The model under review builds one solid part; all positions refer to its coordinate system, in mm. A direction names the side the tool comes from. Round coordinates to 2 decimals unless told otherwise and drop trailing zeros. Loops run counter-clockwise (first coordinate to the right, second up) from the corner with the lowest first, then second, coordinate; pieces in that order, holes last. Notation, with made-up numbers: (77.25, -6.75) - (125.25, -6.75) arc R20 cw to (125.25, 22.25) - close; hole circle Ø7 at (-18, 13.5). An arc over 180 degrees is marked (long way). Answer as CSV lines item,"result".
from build123d import *

# Parameters (mm, degrees)
SKETCH1_W           = 177.8
SKETCH1_H           = 25.4
SKETCH1_W_2         = 167.64
SKETCH1_H_2         = 15.24
BOSS_EXTRUDE2_DEPTH = 25.4
SKETCH3_W           = 193.04
SKETCH3_H           = 39.37
SKETCH3_W_2         = 177.8
SKETCH3_H_2         = 25.4
BOSS_EXTRUDE3_DEPTH = 12.7


with BuildPart() as part:
    # Sketch1 → Boss-Extrude2 (new body)
    with BuildSketch(Plane.XY):
        with Locations((88.9, 12.7)):
            Rectangle(SKETCH1_W, SKETCH1_H)
        with Locations((88.9, 12.7)):
            Rectangle(SKETCH1_W_2, SKETCH1_H_2, mode=Mode.SUBTRACT)
    extrude(amount=BOSS_EXTRUDE2_DEPTH)

    # Sketch3 → Boss-Extrude3 (add)
    with BuildSketch(Plane.XY.offset(25.4)):
        with Locations((88.9, 14.605)):
            Rectangle(SKETCH3_W, SKETCH3_H)
        with Locations((88.9, 12.7)):
            Rectangle(SKETCH3_W_2, SKETCH3_H_2, mode=Mode.SUBTRACT)
    extrude(amount=-BOSS_EXTRUDE3_DEPTH)


solid = part.part
1. Take a section at A-A (y = 11). State the section outline as (x, z) points, plus the area to 3 significant figures.
Numbers:
outline,"(-7.62, 12.7) - (0, 12.7) - (0, 0) - (5.08, 0) - (5.08, 25.4) - (-7.62, 25.4) - close; (172.72, 0) - (177.8, 0) - (177.8, 12.7) - (185.42, 12.7) - (185.42, 25.4) - (172.72, 25.4) - close"
area,"452 mm²"
2. Wall thickness on probe 1 along Y at (x, z) = (24, 16.5); probe 2 along X at (y, z) = (11, 20); probe 3 along Y at (x, z) = (158, 8.75): over which ranges is each line inside the solid? List them lowest first.
Numbers:
probe 1,"y = -5.08 to 5.08, 20.32 to 34.29"
probe 2,"x = -7.62 to 5.08, 172.72 to 185.42"
probe 3,"y = 0 to 5.08, 20.32 to 25.4"
3. Take a section at D-D (z = 16.5). State the section outline as (x, y) points, plus the area to 3 significant figures.
Numbers:
outline,"(-7.62, -5.08) - (185.42, -5.08) - (185.42, 34.29) - (-7.62, 34.29) - close; hole (5.08, 5.08) - (172.72, 5.08) - (172.72, 20.32) - (5.08, 20.32) - close"
area,"5,050 mm²"
4. Clearance check with flat-ended pins moving along their axes: pin 1 (4 mm diameter, centred on x = 76, z = 9, fed in from -Y); pin 2 (4 mm diameter, centred on y = 17, z = 6.5, fed in from +X); pin 3 (2 mm diameter, centred on y = 23, z = 5.5, fed in from -X). State where each tip first meets the part, or that it passes through.
Numbers:
pin 1,"stops at y = 0"
pin 2,"stops at x = 177.8"
pin 3,"stops at x = 0"
5. Take a section at C-C (x = 115.5). State the section outline as (y, z) points, plus the area to 3 significant figures.
Numbers:
outline,"(-5.08, 12.7) - (0, 12.7) - (0, 0) - (5.08, 0) - (5.08, 25.4) - (-5.08, 25.4) - close; (20.32, 0) - (25.4, 0) - (25.4, 12.7) - (34.29, 12.7) - (34.29, 25.4) - (20.32, 25.4) - close"
area,"435 mm²"
6. Take a section at B-B (z = 2.75). State the section outline as (x, y) points.
Numbers:
outline,"(0, 0) - (177.8, 0) - (177.8, 25.4) - (0, 25.4) - close; hole (5.08, 5.08) - (172.72, 5.08) - (172.72, 20.32) - (5.08, 20.32) - close"
7. Tool access review of faces 1 (the face through (172.72, 13, 13)), 2 (the face through (177.8, 13, 6)), 3 (the face through (88, 25.4, 6)): name each direction out of +Z, -Z, +X, -X, +Y, -Y from which nothing blocks a thin tool from reaching the whole face with its end or side.
Numbers:
face 1,"+Z, -Z"
face 2,"-Z, +X, +Y, -Y"
face 3,"-Z, +X, -X, +Y"
